Autodesk Inventor part; units mm, degrees
ref_plane "YZ Plane" through (0, 0, 0) normal (1, 0, 0) x (0, 1, 0)
ref_plane "XZ Plane" through (0, 0, 0) normal (0, 1, 0) x (-1, 0, 0)
ref_plane "XY Plane" through (0, 0, 0) normal (0, 0, 1) x (1, 0, 0)
sketch "Эскиз1" plane through (0, 0, 0) normal (1, 0, 0) x (0, 1, 0)
  circle A0 centre (0, 0) radius 5.5
  dimension "d0" = 11
extrude "Выдавливание1" add sketch "Эскиз1" along normal blind 10
sketch "Эскиз2" plane through (10, 0, 0) normal (1, 0, 0) x (0, 0, -1)
  circle A0 centre (0, 0) radius 2.5
  dimension "d3" = 5
extrude "Выдавливание2" cut sketch "Эскиз2" against normal blind 7
sketch "Эскиз3" plane through (0, 0, 0) normal (-1, 0, 0) x (0, 0, 1)
  circle A0 centre (0, 0) radius 1
  dimension "d6" = 2
extrude "Выдавливание3" add sketch "Эскиз3" along normal blind 1
The listing builds one solid part. Answer for the finished solid, in the listing's coordinates (mm). A direction names the side the tool comes from. Coordinates: 2 decimals unless noted, no trailing zeros. Write each loop counter-clockwise with the first axis right and the second up, starting at its lowest first coordinate (ties: lowest second). Pieces come first, ordered by that corner, then holes. Notation, with made-up numbers: (-21.75, 2) - (37.25, 2) arc R32 ccw to (37.25, 36) - close; hole circle Ø5 at (35.5, 67). An arc over 180 degrees is marked (long way). Return JSON: item names as keys, results as strings.
1. The part is cut by section D-D on x = 0.75. Determine the outline of the cut face in (y, z), then the cut area to 3 significant figures.
Final values:
{"outline": "circle Ø11 at (0, 0)", "area": "95.0 mm^2"}
2. The part is cut by section A-A on z = 0. Determine the outline of the cut face in (x, y).
Final values:
{"outline": "(-1, -1) - (0, -1) - (0, -5.5) - (10, -5.5) - (10, -2.5) - (3, -2.5) - (3, 2.5) - (10, 2.5) - (10, 5.5) - (0, 5.5) - (0, 1) - (-1, 1) - close"}
3. Consider line 1 along X through (y, z) = (5, -0.5); line 2 along Y through (x, z) = (4.75, -0.75); line 3 along Z through (x, y) = (5, 0.25). Determine where each line is inside the solid, lowest interval first.
Final values:
{"line 1": "0 to 10", "line 2": "-5.45 to -2.38, 2.38 to 5.45", "line 3": "-5.49 to -2.49, 2.49 to 5.49"}
4. Which of the six approach directions +Z, -Z, +X, -X, +Y, -Y give full straight-line access (tool end or side, diameter ignored) to faces 5 (the face through (-0.493, 0.976, -0.217)), 6 (the face through (10, -3, 0))?
Final values:
{"face 5": "-X", "face 6": "+Z, -Z, +X, +Y, -Y"}
5. Each of these flat-tipped pins is pushed along its axis until it touches: pin 1 Ø5.5 at (y, z) = (2.5, 2) entering from -X; pin 2 Ø4 at (x, y) = (7.5, -3) entering from -Z; pin 3 Ø2 at (y, z) = (3, 2) entering from -X; pin 4 Ø1 at (x, z) = (6, 3) entering from +Y. Where does it stop, or does it pass through?
Final values:
{"pin 1": "x = -1", "pin 2": "z = -5.41", "pin 3": "x = 0", "pin 4": "y = 4.9"}
6. The part is cut by section C-C on x = 9.25. Determine the outline of the cut face in (y, z).
Final values:
{"outline": "circle Ø11 at (0, 0); hole circle Ø5 at (0, 0)"}
7. For a pull along Y with two mould halves and no side action, classify faces 1 (the face through (-1, 0, 0)), 2 (the face through (3, 0, 0)), 3 (the face through (6.55, -2.44, 0.54)), 4 (the face through (4.93, -1.19, 5.37)) as +Y half, -Y half, draft (parallel to the pull), parting line (faces both ways), or undercut.
Final values:
{"face 1": "draft", "face 2": "undercut", "face 3": "undercut", "face 4": "parting line"}
